Input: part model. Units: mm. Frame: model coordinates. A direction names the side the tool comes from. Coordinates: 2 decimals unless noted, no trailing zeros. Write each loop counter-clockwise with the first axis right and the second up, starting at its lowest first coordinate (ties: lowest second). Pieces come first, ordered by that corner, then holes.
from build123d import *

# Parameters (mm, degrees)
F0_W     = 300
F0_H     = 160
F1_DEPTH = 25
F2_R     = 23.600051
F3_DEPTH = 25.001
F5_DEPTH = 25.001
F7_DEPTH = 25.001


with BuildPart() as f1:
    # F0 (on Front) → F1 (new body)
    with BuildSketch(Plane.XZ):
        with Locations((-34.793959, -40.223419)):
            Rectangle(F0_W, F0_H)
    extrude(amount=F1_DEPTH)

    # F2 (on face) → F3 (cut, through all)
    with BuildSketch(Plane.XZ.offset(25)):
        with Locations((-154.207721, 8.238197)):
            Circle(F2_R)
        with Locations((-42, 7)):
            Circle(F2_R)
        with Locations((70.207721, 5.761803)):
            Circle(F2_R)
        with Locations((73.415443, -82.476395)):
            Circle(F2_R)
        with Locations((-38.792279, -81.238197)):
            Circle(F2_R)
        with Locations((-151, -80)):
            Circle(F2_R)
    extrude(amount=-F3_DEPTH, mode=Mode.SUBTRACT)

    # F4 (on face) → F5 (cut, through all)
    with BuildSketch(Plane.XZ.offset(25)):
        Polygon((-86.684604, -44.342975), (-99.012743, -25.174466), (-121.777227, -26.266693), (-132.213573, -46.527428), (-119.885435, -65.695936), (-97.12095, -64.60371), align=None)
    extrude(amount=-F5_DEPTH, mode=Mode.SUBTRACT)

    # F6 (on face) → F7 (cut, through all)
    with BuildSketch(Plane.XZ.offset(25)):
        Polygon((36.027657, -52.399745), (21.085804, -26.581729), (-8.085875, -32.814069), (-11.173111, -62.483884), (16.090551, -74.588498), align=None)
    extrude(amount=-F7_DEPTH, mode=Mode.SUBTRACT)


solid = f1.part
Item 1: Section query C-C, the plane y = -11.5. State how many separate pieces and enclosed holes the cut face has, then the cut area to 3 significant figures.
Item 2: Section query B-B, the plane z = -88.5. Return loops of the section in (x, y).
Item 3: Section query D-D, the plane x = -150.5. Return loops of the section in (y, z).
Item 4: Pull-direction query (Z, two-part tool) for faces 1 (the face through (25.92, -12.68, -63.65)), 2 (the face through (-37, -12, 39.777)), 3 (the face through (-184.794, -12, -41)), 4 (the face through (-20.2, -12.68, -2.04)); classes: released by +Z, released by -Z, zero draft, split by the parting line, or undercut.
Item 5: Section query A-A, the plane x = 55. Return loops of the section in (y, z), then the cut area to 3 significant figures.
Item 6: Material intervals for line 1 (Z direction, x = -133, y = -17.5); line 2 (X direction, y = -13.5, z = -76.5); line 3 (X direction, y = -13, z = -48), sorted ascending.
Item 7: Access query for faces 5 (the face through (-92.762, -12.675, -34.893)), 6 (the face through (115.206, -12, -41)). Directions: +Z, -Z, +X, -X, +Y, -Y. A direction counts if a zero-diameter tool reaches every point of the face in a straight line with its end or side. Return the directions, or none.
The answers:
1. separate pieces: 1
1. enclosed holes: 8
1. area: 34,600 mm2
2. outline: (-184.79, -25) - (-173.02, -25) - (-173.02, 0) - (-184.79, 0) - close; (-128.98, -25) - (-61.25, -25) - (-61.25, 0) - (-128.98, 0) - close; (-16.34, -25) - (50.6, -25) - (50.6, 0) - (-16.34, 0) - close; (96.23, -25) - (115.21, -25) - (115.21, 0) - (96.23, 0) - close
3. outline: (-25, -120.22) - (0, -120.22) - (0, -103.59) - (-25, -103.59) - close; (-25, -56.41) - (0, -56.41) - (0, -15.07) - (-25, -15.07) - close; (-25, 31.55) - (0, 31.55) - (0, 39.78) - (-25, 39.78) - close
4. face 1: undercut
4. face 2: released by +Z
4. face 3: zero draft
4. face 4: undercut
5. outline: (-25, -120.22) - (0, -120.22) - (0, -97.24) - (-25, -97.24) - close; (-25, -67.72) - (0, -67.72) - (0, -12.29) - (-25, -12.29) - close; (-25, 23.81) - (0, 23.81) - (0, 39.78) - (-25, 39.78) - close
5. area: 2,360 mm2
6. line 1: z = -120.22 to -95.26, -64.74 to -2.12, 18.59 to 39.78
6. line 2: x = -184.79 to -174.34, -127.66 to -61.91, -15.67 to 50.58, 96.25 to 115.21
6. line 3: x = -184.79 to -131.27, -88.57 to -9.67, 33.48 to 115.21
7. face 5: +Y, -Y
7. face 6: +Z, -Z, +X, +Y, -Y
